from build123d import *

# Parameters (mm, degrees)
EXTRUDE_1_DEPTH = 5
SCALE_1_SCALE   = 0.6


with BuildPart() as part:
    # Эскиз1 → Бобышка-Вытянуть1 (new body)
    with BuildSketch(Plane.XY):
        with BuildLine():
            Line((5, 29.434281034), (7.5, 78.684281034))
            ThreePointArc((7.5, 78.684281034), (5.562430401, 89.290882752), (0, 98.527415867))
            ThreePointArc((0, 98.527415867), (-5.562430401, 89.290882752), (-7.5, 78.684281034))
            Line((-7.5, 78.684281034), (-5, 29.434281034))
            ThreePointArc((-5, 29.434281034), (-8.525159088, 2.45546227), (-18.863936417, -22.711839767))
            ThreePointArc((-18.863936417, -22.711839767), (-34.990467135, -15.25225811), (-19.576058944, -6.414477187))
            Line((-19.576058944, -6.414477187), (-22.449472465, 34.677250594))
            ThreePointArc((-22.449472465, 34.677250594), (-33.881518529, 67.398455427), (-60, 90.184281034))
            Line((-60, 90.184281034), (-60, -59.815718966))
            Line((-60, -59.815718966), (-27.583269132, -59.815718966))
            ThreePointArc((-27.583269132, -59.815718966), (-20.06001769, -79.093095091), (-5.945767968, -94.225989636))
            ThreePointArc((-5.945767968, -94.225989636), (-2.542345747, -97.496033993), (0, -101.472584133))
            ThreePointArc((0, -101.472584133), (2.542345747, -97.496033993), (5.945767968, -94.225989636))
            ThreePointArc((5.945767968, -94.225989636), (20.06001769, -79.093095091), (27.583269132, -59.815718966))
            Line((27.583269132, -59.815718966), (60, -59.815718966))
            Line((60, -59.815718966), (60, 90.184281034))
            ThreePointArc((60, 90.184281034), (33.881518529, 67.398455427), (22.449472466, 34.677250594))
            Line((22.449472466, 34.677250594), (19.576058945, -6.414477187))
            ThreePointArc((19.576058945, -6.414477187), (34.990467135, -15.25225811), (18.863936417, -22.711839767))
            ThreePointArc((18.863936417, -22.711839767), (8.525159088, 2.45546227), (5, 29.434281034))
        make_face()
        with BuildLine():
            Line((18.5, -49.815718966), (4.5, -49.815718966))
            ThreePointArc((4.5, -49.815718966), (7.858362699, -40.718710911), (16.322222222, -35.986138931))
            ThreePointArc((16.322222222, -35.986138931), (17.952221542, -42.815718966), (18.5, -49.815718966))
        make_face(mode=Mode.SUBTRACT)
        with BuildLine():
            Line((5, -59.815718966), (17.374821937, -59.815718966))
            ThreePointArc((17.374821937, -59.815718966), (12.779082294, -71.773717375), (5, -81.952146894))
            Line((5, -81.952146894), (5, -59.815718966))
        make_face(mode=Mode.SUBTRACT)
        with BuildLine():
            Line((28.5, -49.815718966), (50, -49.815718966))
            Line((50, -49.815718966), (50, -19.815718966))
            Line((50, -19.815718966), (44.364916731, -19.815718966))
            ThreePointArc((44.364916731, -19.815718966), (37.794087282, -30.18814007), (26.401072965, -34.766583472))
            ThreePointArc((26.401072965, -34.766583472), (27.972740949, -42.218318526), (28.5, -49.815718966))
        make_face(mode=Mode.SUBTRACT)
        with BuildLine():
            Line((44.364916731, -9.815718966), (50, -9.815718966))
            Line((50, -9.815718966), (50, 71.093478113))
            ThreePointArc((50, 71.093478113), (37.591425702, 53.700101468), (32.355603325, 32.985651651))
            Line((32.355603325, 32.985651651), (30.360374841, 4.452554998))
            ThreePointArc((30.360374841, 4.452554998), (39.273434111, -0.806112309), (44.364916731, -9.815718966))
        make_face(mode=Mode.SUBTRACT)
        with BuildLine():
            Line((-44.364916731, -19.815718966), (-50, -19.815718966))
            Line((-50, -19.815718966), (-50, -49.815718966))
            Line((-50, -49.815718966), (-28.5, -49.815718966))
            ThreePointArc((-28.5, -49.815718966), (-27.972740949, -42.218318526), (-26.401072965, -34.766583472))
            ThreePointArc((-26.401072965, -34.766583472), (-37.794087282, -30.18814007), (-44.364916731, -19.815718966))
        make_face(mode=Mode.SUBTRACT)
        with BuildLine():
            Line((-5, -81.952146894), (-5, -59.815718966))
            Line((-5, -59.815718966), (-17.374821937, -59.815718966))
            ThreePointArc((-17.374821937, -59.815718966), (-12.779082294, -71.773717375), (-5, -81.952146894))
        make_face(mode=Mode.SUBTRACT)
        with BuildLine():
            Line((-50, -9.815718966), (-50, 71.093478113))
            ThreePointArc((-50, 71.093478113), (-37.591425702, 53.700101468), (-32.355603325, 32.985651651))
            Line((-32.355603325, 32.985651651), (-30.360374841, 4.452554998))
            ThreePointArc((-30.360374841, 4.452554998), (-39.273434111, -0.806112309), (-44.364916731, -9.815718966))
            Line((-44.364916731, -9.815718966), (-50, -9.815718966))
        make_face(mode=Mode.SUBTRACT)
        with BuildLine():
            Line((-18.5, -49.815718966), (-4.5, -49.815718966))
            ThreePointArc((-4.5, -49.815718966), (-7.858362699, -40.718710911), (-16.322222222, -35.986138931))
            ThreePointArc((-16.322222222, -35.986138931), (-17.952221542, -42.815718966), (-18.5, -49.815718966))
        make_face(mode=Mode.SUBTRACT)
        with BuildLine():
            ThreePointArc((11.091351129, -26.987842983), (5.008387109, -29.966880672), (0, -34.526834114))
            ThreePointArc((0, -34.526834114), (-5.008387109, -29.966880672), (-11.091351129, -26.987842983))
            ThreePointArc((-11.091351129, -26.987842983), (-4.677676581, -13.850648093), (0, 0))
            ThreePointArc((0, 0), (4.677676581, -13.850648093), (11.091351129, -26.987842983))
        make_face(mode=Mode.SUBTRACT)
    extrude(amount=EXTRUDE_1_DEPTH)


with BuildPart() as part_1:
    # Масштаб1: scaled about (0, -2.486348983, 2.5)
    add(part.part.scale(SCALE_1_SCALE).moved(Location((0, -0.994539593, 1))))


solid = part_1.part
Read the model definition and answer for the solid it produces. Units are mm, in the model's axes. A direction names the side the tool comes from. Round coordinates to 2 decimals unless told otherwise and drop trailing zeros. Write each loop counter-clockwise with the first axis right and the second up, starting at its lowest first coordinate (ties: lowest second). Pieces come first, ordered by that corner, then holes. Notation, with made-up numbers: M 26.25,54 L 84.25,54 A29 ccw 84.25,84 Z; hole C 33,12.5 d2. An arc over 180 degrees is marked long. Use a Markdown table: item, result.
1) For a pull along X with two mould halves and no side action, classify faces 4 (the flat face through (18.823, 10.357, 2.479)), 5 (the flat face through (26, -36.884, 2)) as pulls with the +X half, pulls with the -X half, needs draft (parallel to the pull), parting line crosses it, or undercut.
Answers follow:
| item | result |
|---|---|
| face 4 | undercut |
| face 5 | needs draft |
2) A tool of negligible diameter and unlimited length cuts with its end or side. For faces 1 (the flat face through (-26, -36.884, 2)), 2 (the flat face through (30, -22, 2)), 3 (the cylindrical face through (-20.165, 39.2, 2.479)), from which of +Z, -Z, +X, -X, +Y, -Y can it reach the whole face along a straight path? Write none if from no direction.
Answers follow:
| item | result |
|---|---|
| face 1 | +Z, -Z, -X, -Y |
| face 2 | +Z, -Z |
| face 3 | +Z, -Z, +Y |
3) The part is cut by section A-A (x = -8.5). Write down the section's boundary in (y, z).
Answers follow:
| item | result |
|---|---|
| outline | M -53.1,1 L -42.44,1 L -42.44,4 L -53.1,4 Z; M -36.88,1 L -30.88,1 L -30.88,4 L -36.88,4 Z; M -22.9,1 L -9.08,1 L -9.08,4 L -22.9,4 Z |
4) Flat-ended cylindrical pins translate along their axes: pin 1 (0.9 mm diameter, centred on x = 28, z = 2.5, fed in from +Y); pin 2 (0.9 mm diameter, centred on x = -28.5, z = 2, fed in from -Y); pin 3 (0.9 mm diameter, centred on x = 22, z = 2, fed in from +Y). Find the tip coordinate at first contact, or state that the pin passes through.
Answers follow:
| item | result |
|---|---|
| pin 1 | stops at y = 48.29 |
| pin 2 | stops at y = -36.88 |
| pin 3 | stops at y = 42.3 |
5) The part is cut by section B-B (y = -48). Write down the section's boundary in (x, z), plus the area to 3 significant figures.
Answers follow:
| item | result |
|---|---|
| outline | M -12.31,1 L -4.98,1 L -4.98,4 L -12.31,4 Z; M -3,1 L 3,1 L 3,4 L -3,4 Z; M 4.98,1 L 12.31,1 L 12.31,4 L 4.98,4 Z |
| area | 62.0 mm2 |
6) The part is cut by section C-C (y = 37). Write down the section's boundary in (x, z), plus the area to 3 significant figures.
Answers follow:
| item | result |
|---|---|
| outline | M -36,1 L -30,1 L -30,4 L -36,4 Z; M -25.94,1 L -18.8,1 L -18.8,4 L -25.94,4 Z; M -4.03,1 L 4.03,1 L 4.03,4 L -4.03,4 Z; M 18.8,1 L 25.94,1 L 25.94,4 L 18.8,4 Z; M 30,1 L 36,1 L 36,4 L 30,4 Z |
| area | 103 mm2 |
7) The part is cut by section D-D (z = 1.8). Give the number of separate pieces and of enclosed holes in the cut face, plus the area to 3 significant figures.
Answers follow:
| item | result |
|---|---|
| separate pieces | 1 |
| enclosed holes | 9 |
| area | 3,730 mm2 |
8) Straight lines are drawn through the part: line 1 along X through (y, z) = (12, 2.05); line 2 along X through (y, z) = (-17, 2.45); line 3 along X through (y, z) = (48, 2.05). For each, find the intervals that lie inside material, in ascending order. Write a range as [from, to].
Answers follow:
| item | result |
|---|---|
| line 1 | x = [-36, -30], [-18.94, -12.92], [-3.17, 3.17], [12.92, 18.94], [30, 36] |
| line 2 | x = [-36, -30], [-24.66, -6.55], [6.55, 24.66], [30, 36] |
| line 3 | x = [-36, -28.1], [-4.41, 4.41], [28.1, 36] |
